from build123d import *

# Parameters (mm, degrees)
SKETCH1_W           = 26
SKETCH1_H           = 26
BOSS_EXTRUDE1_DEPTH = 4.5
FILLET1_R           = 2
SKETCH2_W           = 18
SKETCH2_H           = 18
CUT_EXTRUDE1_DEPTH  = 0.25
SKETCH3_R           = 0.95
BOSS_EXTRUDE2_DEPTH = 1.5


with BuildPart() as part:
    # Sketch1 → Boss-Extrude1 (new, symmetric)
    with BuildSketch(Plane.XY):
        Rectangle(SKETCH1_W, SKETCH1_H)
    extrude(amount=BOSS_EXTRUDE1_DEPTH, both=True)

    # Fillet1
    fillet1_edges = [part.edges().sort_by_distance(p)[0] for p in [
        (-13, 13, 0),
        (13, 13, 0),
        (13, -13, 0),
        (-13, -13, 0),
    ]]
    fillet(fillet1_edges, radius=FILLET1_R)

    # Sketch2 → Cut-Extrude1 (cut, symmetric)
    with BuildSketch(Plane.XY.offset(4.5)):
        Rectangle(SKETCH2_W, SKETCH2_H)
    extrude(amount=CUT_EXTRUDE1_DEPTH, both=True, mode=Mode.SUBTRACT)

    # Sketch3 → Boss-Extrude2 (add, symmetric)
    with BuildSketch(Plane(origin=(0, 0, -4.5), x_dir=(-1, 0, 0), z_dir=(0, 0, -1))):
        with Locations(Location((-9, 0, 0), (0, 0, 180))):
            Circle(SKETCH3_R)
        with Locations(Location((9, 0, 0), (0, 0, 180))):
            Circle(SKETCH3_R)
    extrude(amount=BOSS_EXTRUDE2_DEPTH, both=True)


solid = part.part
Source: CAD feature listing. Evaluate the final solid. Frame: model axes, mm. A direction names the side the tool comes from. Coordinates: 2 decimals unless noted, no trailing zeros. Loops run counter-clockwise (first coordinate to the right, second up) from the corner with the lowest first, then second, coordinate; pieces in that order, holes last. Notation, with made-up numbers: M 27.25,71.25 L 82.25,71.25 A32 ccw 82.25,108.25 Z; hole C 66.25,-31.5 d7. An arc over 180 degrees is marked long. Answer in a Markdown table with one row per item.
Q1. Section C-C on x = 10.5. Return the cut outline in (y, z).
Answers below:
| item | result |
|---|---|
| outline | M -13,-4.5 L 13,-4.5 L 13,4.5 L -13,4.5 Z |
Q2. Set-up query: faces 4 (the flat face through (-12, 0, 4.5)), 5 (the cylindrical face through (-9.95, -0.04, -5.26)), 6 (the flat face through (0, 0, 4.25)). Return all of +Z, -Z, +X, -X, +Y, -Y with unobstructed straight access to the full face (end or side cutting, diameter ignored); none if empty.
Answers below:
| item | result |
|---|---|
| face 4 | +Z, +X, -X, +Y, -Y |
| face 5 | -Z |
| face 6 | +Z |
Q3. Ray query, probe 1 along Z at (x, y) = (5.5, 1); probe 2 along Z at (x, y) = (-10, -11.25); probe 3 along Y at (x, z) = (12, -1.25). Return the intervals inside material, ascending. Write a range as from..to.
Answers below:
| item | result |
|---|---|
| probe 1 | z = -4.5..4.25 |
| probe 2 | z = -4.5..4.5 |
| probe 3 | y = -12.73..12.73 |
Q4. Section A-A on y = 0. Return the cut outline in (x, z), plus the area to 3 significant figures.
Answers below:
| item | result |
|---|---|
| outline | M -13,-4.5 L -9.95,-4.5 L -9.95,-6 L -8.05,-6 L -8.05,-4.5 L 8.05,-4.5 L 8.05,-6 L 9.95,-6 L 9.95,-4.5 L 13,-4.5 L 13,4.5 L 9,4.5 L 9,4.25 L -9,4.25 L -9,4.5 L -13,4.5 Z |
| area | 235 mm^2 |
Q5. Section B-B on x = 6. Return the cut outline in (y, z), plus the area to 4 significant figures.
Answers below:
| item | result |
|---|---|
| outline | M -13,-4.5 L 13,-4.5 L 13,4.5 L 9,4.5 L 9,4.25 L -9,4.25 L -9,4.5 L -13,4.5 Z |
| area | 229.5 mm^2 |
Q6. First-contact query: pin 1 (3 mm diameter, centred on x = -6.5, y = -7.5, fed in from -Z). Flat tip, straight axial feed; report the tip coordinate or a pass-through.
Answers below:
| item | result |
|---|---|
| pin 1 | stops at z = -4.5 |
Q7. Draft query along X for faces 1 (the flat face through (9, 0, -6)), 2 (the flat face through (-13, 0, 0)), 3 (the cylindrical face through (8.05, -0.04, -5.24)). Return one class per face: pulls with the +X half, pulls with the -X half, needs draft (parallel to the pull), parting line crosses it, or undercut.
Answers below:
| item | result |
|---|---|
| face 1 | needs draft |
| face 2 | pulls with the -X half |
| face 3 | undercut |
